Here's how the part is built. I have some questions about the finished solid (model axes, mm). Coordinates: 2 decimals unless noted, no trailing zeros. Write each loop counter-clockwise with the first axis right and the second up, starting at its lowest first coordinate (ties: lowest second). Pieces come first, ordered by that corner, then holes.
Item 1: I'm going to push flat-ended pins straight in: P1, Ø3.5, axis at x = 10, y = 7.5, coming from the +Z side; P2, Ø3, axis at y = 2.5, z = 2.5, coming from the -X side; P3, Ø1.5, axis at y = 2.5, z = -2.5, coming from the -X side. Where does each tip first touch, or does it pass through?
Item 2: I want a section at D-D (z = 25.5). Please give me the cut outline in (x, y), and give its area (3 significant figures).
Item 3: I want a section at B-B (z = 17). Please give me the cut outline in (x, y).
Item 4: Please list where these lines run through material, in increasing order: line 1 (Z direction, x = 12, y = 8); line 2 (Y direction, x = 10, z = 28.25); line 3 (X direction, y = 6, z = 0).
Item 5: I want a section at A-A (x = 4.25). Please give me the cut outline in (y, z), and give its area (3 significant figures).
Item 6: I want a section at C-C (y = 7.5). Please give me the cut outline in (x, z), and give its area (3 significant figures).
from build123d import *

# Parameters (mm, degrees)
EXTRUDE_1_DEPTH     = 15
SKETCH_3_R          = 2
CUT_EXTRUDE_3_DEPTH = 61
SKETCH_5_R          = 3
CUT_EXTRUDE_4_DEPTH = 17
CUT_EXTRUDE_START   = 17
SKETCH_6_R          = 3
CUT_EXTRUDE_5_DEPTH = 17


with BuildPart() as part:
    # Эскиз1 → Вытянуть1 (new body)
    with BuildSketch(Plane(origin=(0, 0, 0), x_dir=(1, 0, 0), z_dir=(0, 1, 0))):
        with BuildLine():
            Line((0, -14), (0, -38))
            Line((0, -38), (20.00009991, -38))
            Line((20.00009991, -38), (20.00009991, 38))
            Line((20.00009991, 38), (0, 38))
            Line((0, 38), (0, 14))
            ThreePointArc((0, 14), (14, 0), (0, -14))
        make_face()
    extrude(amount=EXTRUDE_1_DEPTH)

    # Эскиз3 → Вырез-Вытянуть3 (cut, symmetric)
    with BuildSketch(Plane(origin=(20.00009991, 0, 0), x_dir=(0, 0, -1), z_dir=(1, 0, 0))):
        with Locations((-17, 7.5)):
            Circle(SKETCH_3_R)
        with Locations((17, 7.5)):
            Circle(SKETCH_3_R)
    extrude(amount=CUT_EXTRUDE_3_DEPTH, both=True, mode=Mode.SUBTRACT)

    # Эскиз5 → Вырез-Вытянуть4 (cut)
    with BuildSketch(Plane.XY.offset(38)):
        with Locations((10, 7.5)):
            Circle(SKETCH_5_R)
    extrude(amount=-CUT_EXTRUDE_4_DEPTH, mode=Mode.SUBTRACT)

    # Эскиз6 → Вырез-Вытянуть5 (cut)
    with BuildSketch(Plane.XY.offset(-38).offset(CUT_EXTRUDE_START)):
        with Locations((10, 7.5)):
            Circle(SKETCH_6_R)
    extrude(amount=-CUT_EXTRUDE_5_DEPTH, mode=Mode.SUBTRACT)


solid = part.part
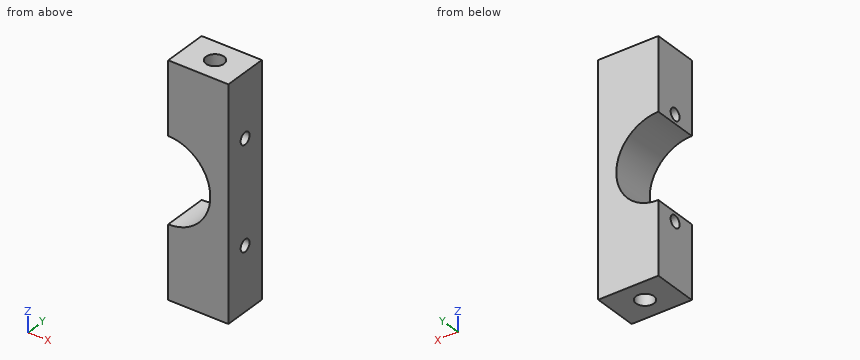
Answer:
1. P1: stops at z = 21
1. P2: stops at x = 13.42
1. P3: stops at x = 13.62
2. outline: (0, 0) - (20, 0) - (20, 15) - (0, 15) - close; hole circle Ø6 at (10, 7.5)
2. area: 272 mm2
3. outline: (0, 0) - (20, 0) - (20, 5.5) - (0, 5.5) - close; (0, 9.5) - (20, 9.5) - (20, 15) - (0, 15) - close
4. line 1: z = -21 to -18.94, -15.06 to -7.21, 7.21 to 15.06, 18.94 to 21
4. line 2: y = 0 to 4.5, 10.5 to 15
4. line 3: x = 14 to 20
5. outline: (0, -38) - (15, -38) - (15, -13.34) - (0, -13.34) - close; (0, 13.34) - (15, 13.34) - (15, 38) - (0, 38) - close; hole circle Ø4 at (7.5, -17); hole circle Ø4 at (7.5, 17)
5. area: 715 mm2
6. outline: (0, -38) - (7, -38) - (7, -21) - (13, -21) - (13, -38) - (20, -38) - (20, -19) - (0, -19) - close; (0, -15) - (20, -15) - (20, 15) - (0, 15) - (0, 14) arc R14 cw to (0, -14) - close; (0, 19) - (20, 19) - (20, 38) - (13, 38) - (13, 21) - (7, 21) - (7, 38) - (0, 38) - close
6. area: 848 mm2
